from build123d import *

# Parameters (mm, degrees)
F1_DEPTH      = 3.302
F2_DEPTH      = 6.35
F3_T1_DEPTH   = 4.6338919233
F4_T1_DEPTH   = 4.4582047696
F5_R          = 1.397
F6_DEPTH      = 6.351
F6_DEPTH_BACK = 25.4
F7_R          = 3.81
F8_DEPTH      = 5.842
F9_T1_DEPTH   = 8.456355204
F9_T3_DEPTH   = 2.54


# Not quite as in the source:
# - a fillet or chamfer that OpenCascade refuses, or shapes differently, is made with other operations: its cross-section is extruded or revolved along the edge and cut away or added


with BuildPart() as f1:
    # F0 (on Top) → F1 (new body)
    with BuildSketch(Plane.XY):
        with BuildLine():
            Line((0.8864303251, 2.1758656964), (4.1494522244, 10.1854037464))
            ThreePointArc((4.1494522244, 10.1854037464), (-0.7354841661, 10.9735803766), (-5.4715498037, 9.5405736717))
            Line((-5.4715498037, 9.5405736717), (-1.1688645655, 2.0381133132))
            ThreePointArc((-1.1688645655, 2.0381133132), (-0.157118442, 2.3442406116), (0.8864303251, 2.1758656964))
        make_face()
    extrude(amount=F1_DEPTH)



with BuildPart() as f1b:
    # F0 (on Top) → F1, piece 2 (new body)
    with BuildSketch(Plane.XY):
        with BuildLine():
            Line((-2.3275701308, -0.320261668), (-10.8955445044, -1.4991708351))
            ThreePointArc((-10.8955445044, -1.4991708351), (-9.1356572935, -6.1237381602), (-5.5266042645, -9.5087879639))
            Line((-5.5266042645, -9.5087879639), (-1.1806256223, -2.0313230639))
            ThreePointArc((-1.1806256223, -2.0313230639), (-1.9516127013, -1.3081888679), (-2.3275701308, -0.320261668))
        make_face()
    extrude(amount=F1_DEPTH)


with BuildPart() as f1c:
    # F0 (on Top) → F1, piece 3 (new body)
    with BuildSketch(Plane.XY):
        with BuildLine():
            ThreePointArc((6.74609228, -8.6862329113), (9.8711414597, -4.8498422164), (10.9981540682, -0.0317857078))
            Line((10.9981540682, -0.0317857078), (2.3494901878, -0.0067902494))
            ThreePointArc((2.3494901878, -0.0067902494), (2.1087311432, -1.0360517437), (1.4411398058, -1.8556040284))
            Line((1.4411398058, -1.8556040284), (6.74609228, -8.6862329113))
        make_face()
    extrude(amount=F1_DEPTH)


with BuildPart() as f1_1:
    add(f1.part)

    add(f1b.part)  # F2 merges F1b

    add(f1c.part)  # F2 merges F1c
    # F0 (on Top) → F2 (join)
    with BuildSketch(Plane.XY):
        with BuildLine():
            ThreePointArc((10.9981540682, -0.0317857078), (10.9981885171, -0.0158928705), (10.9982, 0))
            ThreePointArc((10.9982, 0), (9.1267986911, 6.136933183), (4.1494522244, 10.1854037464))
            Line((4.1494522244, 10.1854037464), (0.8864303251, 2.1758656964))
            ThreePointArc((0.8864303251, 2.1758656964), (1.9497202747, 1.3110076661), (2.3495, 0))
            ThreePointArc((2.3495, 0), (2.3494975469, -0.0033951282), (2.3494901878, -0.0067902494))
            Line((2.3494901878, -0.0067902494), (10.9981540682, -0.0317857078))
        make_face()
        with BuildLine():
            Line((0.8864303251, 2.1758656964), (4.1494522244, 10.1854037464))
            ThreePointArc((4.1494522244, 10.1854037464), (-0.7354841661, 10.9735803766), (-5.4715498037, 9.5405736717))
            Line((-5.4715498037, 9.5405736717), (-1.1688645655, 2.0381133132))
            ThreePointArc((-1.1688645655, 2.0381133132), (-0.157118442, 2.3442406116), (0.8864303251, 2.1758656964))
        make_face()
        with BuildLine():
            ThreePointArc((6.74609228, -8.6862329113), (9.8711414597, -4.8498422164), (10.9981540682, -0.0317857078))
            Line((10.9981540682, -0.0317857078), (2.3494901878, -0.0067902494))
            ThreePointArc((2.3494901878, -0.0067902494), (2.1087311432, -1.0360517437), (1.4411398058, -1.8556040284))
            Line((1.4411398058, -1.8556040284), (6.74609228, -8.6862329113))
        make_face()
        with BuildLine():
            Line((-1.1688645655, 2.0381133132), (-5.4715498037, 9.5405736717))
            ThreePointArc((-5.4715498037, 9.5405736717), (-9.8711414597, 4.8498422164), (-10.8955445044, -1.4991708351))
            Line((-10.8955445044, -1.4991708351), (-2.3275701308, -0.320261668))
            ThreePointArc((-2.3275701308, -0.320261668), (-2.1087311432, 1.0360517437), (-1.1688645655, 2.0381133132))
        make_face()
        with BuildLine():
            ThreePointArc((-5.5266042645, -9.5087879639), (0.7354841661, -10.9735803766), (6.74609228, -8.6862329113))
            Line((6.74609228, -8.6862329113), (1.4411398058, -1.8556040284))
            ThreePointArc((1.4411398058, -1.8556040284), (0.157118442, -2.3442406116), (-1.1806256223, -2.0313230639))
            Line((-1.1806256223, -2.0313230639), (-5.5266042645, -9.5087879639))
        make_face()
        with BuildLine():
            Line((-2.3275701308, -0.320261668), (-10.8955445044, -1.4991708351))
            ThreePointArc((-10.8955445044, -1.4991708351), (-9.1356572935, -6.1237381602), (-5.5266042645, -9.5087879639))
            Line((-5.5266042645, -9.5087879639), (-1.1806256223, -2.0313230639))
            ThreePointArc((-1.1806256223, -2.0313230639), (-1.9516127013, -1.3081888679), (-2.3275701308, -0.320261668))
        make_face()
    extrude(amount=-F2_DEPTH)

    # F3: fillet of radius 0.508 on 6 edges, made by hand

    # F3_s2 → F3_t1 (cut)
    with BuildSketch(Plane.XY):
        with BuildLine():
            ThreePointArc((3.9531481969, 9.7035483908), (3.9459668292, 10.1036299064), (3.6513440541, 10.3743958782))
            ThreePointArc((3.6513440541, 10.3743958782), (3.901542663, 10.2829163222), (4.1494522244, 10.1854037464))
            Line((4.1494522244, 10.1854037464), (3.9531481969, 9.7035483908))
        make_face()
        with BuildLine():
            ThreePointArc((10.9837113978, -0.5643466757), (10.8451967866, -0.1889395718), (10.4778487793, -0.0302819762))
            Line((10.4778487793, -0.0302819762), (10.9981540682, -0.0317857078))
            ThreePointArc((10.9981540682, -0.0317857078), (10.9941578867, -0.2981536556), (10.9837113978, -0.5643466757))
        make_face()
        with BuildLine():
            ThreePointArc((-5.212699429, 9.089224208), (-5.2589719244, 9.4866857122), (-5.0031171412, 9.7943464361))
            ThreePointArc((-5.0031171412, 9.7943464361), (-5.2388703034, 9.6702968509), (-5.4715498037, 9.5405736717))
            Line((-5.4715498037, 9.5405736717), (-5.212699429, 9.089224208))
        make_face()
        with BuildLine():
            ThreePointArc((7.1588183524, -8.3493546479), (6.7770167548, -8.4691224698), (6.4269453148, -8.2753009589))
            Line((6.4269453148, -8.2753009589), (6.74609228, -8.6862329113))
            ThreePointArc((6.74609228, -8.6862329113), (6.9544954285, -8.5202932212), (7.1588183524, -8.3493546479))
        make_face()
        with BuildLine():
            ThreePointArc((-5.9805942565, -9.2299997605), (-5.5862248623, -9.2977461404), (-5.2651493503, -9.0589422318))
            Line((-5.2651493503, -9.0589422318), (-5.5266042645, -9.5087879639))
            ThreePointArc((-5.5266042645, -9.5087879639), (-5.7552875833, -9.3721431953), (-5.9805942565, -9.2299997605))
        make_face()
        with BuildLine():
            ThreePointArc((-10.3800935118, -1.428247432), (-10.722983584, -1.6345074366), (-10.8101624065, -2.0250412303))
            ThreePointArc((-10.8101624065, -2.0250412303), (-10.8560380915, -1.762623101), (-10.8955445044, -1.4991708351))
            Line((-10.8955445044, -1.4991708351), (-10.3800935118, -1.428247432))
        make_face()
    extrude(amount=F3_T1_DEPTH, mode=Mode.SUBTRACT)

    # F4: fillet of radius 0.508 on 6 edges, made by hand

    # F4_s2 → F4_t1 (cut)
    with BuildSketch(Plane.XY):
        with BuildLine():
            ThreePointArc((-2.7857353042, -0.3833028373), (-2.4469491553, -0.4559663275), (-2.2335580647, -0.7289503561))
            ThreePointArc((-2.2335580647, -0.7289503561), (-2.2897006824, -0.5267077321), (-2.3275701308, -0.320261668))
            Line((-2.3275701308, -0.320261668), (-2.7857353042, -0.3833028373))
        make_face()
        with BuildLine():
            ThreePointArc((-1.5229431343, -1.7890764264), (-1.3515120564, -2.0901867434), (-1.4130231496, -2.4311741667))
            Line((-1.4130231496, -2.4311741667), (-1.1806256223, -2.0313230639))
            ThreePointArc((-1.1806256223, -2.0313230639), (-1.3572000088, -1.9178525455), (-1.5229431343, -1.7890764264))
        make_face()
        with BuildLine():
            ThreePointArc((-0.7879140674, 2.2134456561), (-1.1343987902, 2.215537146), (-1.3989470146, 2.439301027))
            Line((-1.3989470146, 2.439301027), (-1.1688645655, 2.0381133132))
            ThreePointArc((-1.1688645655, 2.0381133132), (-0.9823090207, 2.1342959584), (-0.7879140674, 2.2134456561))
        make_face()
        with BuildLine():
            ThreePointArc((0.4854895058, 2.2987932029), (0.8285961548, 2.3471032941), (1.0609176577, 2.6041689603))
            Line((1.0609176577, 2.6041689603), (0.8864303251, 2.1758656964))
            ThreePointArc((0.8864303251, 2.1758656964), (0.6887080648, 2.2462928241), (0.4854895058, 2.2987932029))
        make_face()
        with BuildLine():
            ThreePointArc((1.7248176465, -2.220866123), (1.6183530006, -1.8911369665), (1.7480685589, -1.5698428468))
            ThreePointArc((1.7480685589, -1.5698428468), (1.6009926176, -1.719585092), (1.4411398058, -1.8556040284))
            Line((1.4411398058, -1.8556040284), (1.7248176465, -2.220866123))
        make_face()
        with BuildLine():
            ThreePointArc((2.8119701642, -0.0081268603), (2.4859108466, -0.1253504027), (2.3108572018, -0.4243692296))
            ThreePointArc((2.3108572018, -0.4243692296), (2.3395090295, -0.2164434129), (2.3494901878, -0.0067902494))
            Line((2.3494901878, -0.0067902494), (2.8119701642, -0.0081268603))
        make_face()
    extrude(amount=F4_T1_DEPTH, mode=Mode.SUBTRACT)

    # F5 (on face) → F6 (cut, two sides)
    with BuildSketch(Plane.XY) as f6_sk:
        with Locations((-4.4645385024, 6.6395705404)):
            Circle(F5_R)
        with Locations((6.6395705404, 4.4645385024)):
            Circle(F5_R)
        with Locations((4.4645385024, -6.6395705404)):
            Circle(F5_R)
    extrude(amount=-F6_DEPTH, mode=Mode.SUBTRACT)
    extrude(f6_sk.sketch, amount=F6_DEPTH_BACK, mode=Mode.SUBTRACT)

    # F7 (on face) → F8 (cut)
    with BuildSketch(Plane.XY.offset(3.302)):
        with Locations((4.4645385024, -6.6395705404)):
            Circle(F7_R)
        with Locations((6.6395705404, 4.4645385024)):
            Circle(F7_R)
        with BuildLine():
            ThreePointArc((-2.0962074568, 3.6550926868), (-1.0338358569, 4.9823501693), (-0.6545385024, 6.6395705404))
            ThreePointArc((-0.6545385024, 6.6395705404), (-1.5039813545, 9.0377367927), (-3.6735418484, 10.3665564933))
            ThreePointArc((-3.6735418484, 10.3665564933), (-4.3477533155, 10.102348457), (-5.0031171412, 9.7943464361))
            ThreePointArc((-5.0031171412, 9.7943464361), (-5.2589719244, 9.4866857122), (-5.212699429, 9.089224208))
            Line((-5.212699429, 9.089224208), (-4.6049424864, 8.0294970569))
            ThreePointArc((-4.6049424864, 8.0294970569), (-3.5276648091, 7.6758507548), (-3.0675385024, 6.6395705404))
            ThreePointArc((-3.0675385024, 6.6395705404), (-3.1362873981, 6.2067218326), (-3.3357675701, 5.8164756598))
            Line((-3.3357675701, 5.8164756598), (-2.0962074568, 3.6550926868))
        make_face()
        with BuildLine():
            ThreePointArc((-5.0031171412, 9.7943464361), (-4.3477533155, 10.102348457), (-3.6735418484, 10.3665564933))
            ThreePointArc((-3.6735418484, 10.3665564933), (-8.1734837008, 5.7678908314), (-2.0962074568, 3.6550926868))
            Line((-2.0962074568, 3.6550926868), (-3.3357675701, 5.8164756598))
            ThreePointArc((-3.3357675701, 5.8164756598), (-3.1362873981, 6.2067218326), (-3.0675385024, 6.6395705404))
            ThreePointArc((-3.0675385024, 6.6395705404), (-3.5276648091, 7.6758507548), (-4.6049424864, 8.0294970569))
            Line((-4.6049424864, 8.0294970569), (-5.212699429, 9.089224208))
            ThreePointArc((-5.212699429, 9.089224208), (-5.2589719244, 9.4866857122), (-5.0031171412, 9.7943464361))
        make_face()
    extrude(amount=-F8_DEPTH, mode=Mode.SUBTRACT)

    # F9: chamfer of 2.54 on 2 edges, made by hand

    # F9_s2 → F9_t1 (cut)
    with BuildSketch(Plane.XY):
        with BuildLine():
            Line((-1.6990973778, 10.9601467928), (-2.0905864719, 9.5002911113))
            Line((-2.0905864719, 9.5002911113), (-2.1225900483, 9.460839735))
            ThreePointArc((-2.1225900483, 9.460839735), (-2.8366247449, 10.0280040188), (-3.6840884704, 10.3168633472))
            Line((-3.6840884704, 10.3168633472), (-3.6905097091, 10.4144389713))
            ThreePointArc((-3.6905097091, 10.4144389713), (-2.6991406456, 10.7142447599), (-1.7070669555, 11.0103177588))
            Line((-1.7070669555, 11.0103177588), (-1.6990973778, 10.9601467928))
        make_face()
    extrude(amount=F9_T1_DEPTH, mode=Mode.SUBTRACT)

    # F9_s4 → F9_t3 (cut)
    with BuildSketch(Plane.XY.offset(-2.54)):
        with BuildLine():
            Line((-2.0905864719, 9.5002911113), (-1.6990973778, 10.9601467928))
            Line((-1.6990973778, 10.9601467928), (-1.7070669555, 11.0103177588))
            ThreePointArc((-1.7070669555, 11.0103177588), (-2.6991406456, 10.7142447599), (-3.6905097091, 10.4144389713))
            Line((-3.6905097091, 10.4144389713), (-3.6840884704, 10.3168633472))
            ThreePointArc((-3.6840884704, 10.3168633472), (-2.8366247449, 10.0280040188), (-2.1225900483, 9.460839735))
            Line((-2.1225900483, 9.460839735), (-2.0905864719, 9.5002911113))
        make_face()
    extrude(amount=F9_T3_DEPTH, mode=Mode.SUBTRACT)


solid = f1_1.part
The listing builds one solid part. Answer for the finished solid, in the listing's coordinates (mm). A direction names the side the tool comes from. Give positions to 0.01 mm unless a question says otherwise; leave off trailing zeros. Write each loop counter-clockwise with the first axis right and the second up, starting at its lowest first coordinate (ties: lowest second). Pieces come first, ordered by that corner, then holes.
1) Section D-D (z = -5.5) is taken. Count the separate pieces of the cut face and the enclosed holes in it, and give its area (3 significant figures).
2) Section A-A (y = 7) is taken. Write down the section's boundary in (x, z), and give its area (3 significant figures).
3) Section B-B (x = -4.75) is taken. Write down the section's boundary in (y, z), and give its area (3 significant figures).
4) A tool of negligible diameter and unlimited length cuts with its end or side. For faces 4 (the face through (-1.892, 10.239, 0.34)), 5 (the face through (2.487, 6.104, 1.628)), 6 (the face through (-5, 5, -2.54)), from which of +Z, -Z, +X, -X, +Y, -Y can it reach the whole face along a straight path? Write none if from no direction.
5) Given P1, Ø5, axis at x = -7.5, z = -3, coming from the -Y side; P2, Ø4.5, axis at x = -4.46, y = 6.64, coming from the +Z side; P3, Ø1, axis at y = -6, z = 1.5, coming from the -X side, each flat-ended and moving along its own axis, determine where each tip first touches the part or whether it passes through.
6) Find the intervals of material crossed by L1, parallel to Y at x = 1.75, z = -1; L2, parallel to Z at x = 0.5, y = -7.75; L3, parallel to Y at x = -1, z = -4, in increasing order.
7) For a pull along Y with two mould halves and no side action, classify faces 1 (the face through (-1, -7, 0)), 2 (the face through (6.227, -3.262, -0.227)), 3 (the face through (-6.53, -0.9, 1.63)) as pulls with the +Y half, pulls with the -Y half, needs draft (parallel to the pull), parting line crosses it, or undercut.
8) Section C-C (z = 2.5) is taken. Write down the section's boundary in (x, y).
Response:
1. separate pieces: 1
1. enclosed holes: 4
1. area: 344 mm2
2. outline: (-8.48, -6.35) - (-5.81, -6.35) - (-5.81, -2.54) - (-8.26, -2.54) - (-8.26, 0) - (-8.48, 0) - close; (-3.11, -6.35) - (8.48, -6.35) - (8.48, -2.54) - (3.8, -2.54) - (3.8, 0) - (2.85, 0) - (2.85, 3.3) - (-0.67, 3.3) - (-0.67, -2.54) - (-3.11, -2.54) - close
2. area: 77.9 mm2
3. outline: (-9.92, -6.35) - (5.27, -6.35) - (5.27, -2.54) - (2.84, -2.54) - (2.84, 0) - (-0.65, 0) - (-0.65, 3.3) - (-8.17, 3.3) - (-8.17, 0) - (-9.92, 0) - close; (8.01, -6.35) - (9.92, -6.35) - (9.92, -2.54) - (8.01, -2.54) - close
3. area: 122 mm2
4. face 4: +Z, -X, +Y
4. face 5: +Z, +X
4. face 6: +Z
5. P1: stops at y = -9.8
5. P2: stops at z = -2.54
5. P3: stops at x = -9.52
6. L1: y = -10.86 to -9.31, -3.97 to -1.57, 1.57 to 10.86
6. L2: z = -6.35 to 0
6. L3: y = -10.95 to -2.13, 2.13 to 10.95
7. face 1: needs draft
7. face 2: undercut
7. face 3: pulls with the +Y half
8. outline: (-10.81, -2.03) arc R11 ccw to (-5.98, -9.23) arc R0.51 ccw to (-5.27, -9.06) - (-1.41, -2.43) arc R0.51 ccw to (-1.52, -1.79) arc R2.35 cw to (-2.23, -0.73) arc R0.51 ccw to (-2.79, -0.38) - (-10.38, -1.43) arc R0.51 ccw to start; (-2.1, 3.66) - (-1.4, 2.44) arc R0.51 ccw to (-0.79, 2.21) arc R2.35 cw to (0.49, 2.3) arc R0.51 ccw to (1.06, 2.6) - (3.95, 9.7) arc R0.51 ccw to (3.65, 10.37) arc R11 ccw to (-1.73, 10.86) - (-2.06, 9.6) arc R3.81 cw to start; (1.72, -2.22) - (2.58, -3.33) arc R3.81 cw to (8.21, -7.31) arc R11 ccw to (10.98, -0.56) arc R0.51 ccw to (10.48, -0.03) - (2.81, -0.01) arc R0.51 ccw to (2.31, -0.42) arc R2.35 cw to (1.75, -1.57) arc R0.51 ccw to start
